Part print with two shaded views. Sizes in mm from the minimum x, y, z corner. A direction names the side the tool comes from. Round coordinates to 2 decimals unless told otherwise and drop trailing zeros. Write each loop counter-clockwise with the first axis right and the second up, starting at its lowest first coordinate (ties: lowest second). Pieces come first, ordered by that corner, then holes. Notation, with made-up numbers: (11.5, 48.5) -> (15.5, 48.5) arc R26 cw to (15.5, 73.5) -> close; hole circle Ø8 at (26, 30). An arc over 180 degrees is marked (long way). Return JSON: item names as keys, results as strings. Group by question number.
(1) Saw through at A-A (x = 5). List the corners of the cut face in (y, z).
(2) Saw through at C-C (z = 17.35). List the corners of the cut face in (x, y), plus the area to 3 significant figures.
(3) Saw through at D-D (x = 18). List the corners of the cut face in (y, z).
(4) Saw through at B-B (z = 3.1). List the corners of the cut face in (x, y), plus the area to 3 significant figures.
(5) Drop flat-ended pins along their axis: pin 1 Ø10 at (x, z) = (15.5, 30.5) entering from +Y; pin 2 Ø8 at (y, z) = (23, 27.5) entering from -X; pin 3 Ø4 at (x, y) = (10, 33.5) entering from +Z; pin 4 Ø3.5 at (x, z) = (10, 5) entering from +Y. Give the stop position or say it passes through.
(6) Drill centre lines: L1, parallel to Z at x = 5, y = 28.25; L2, parallel to X at y = 28, z = 51; L3, parallel to Y at x = 16.5, z = 16.5. Where is each one in solid material? Low to high. Write a range as from..to.
(7) Tool access for the marked faces 1, 2 and 3: list every direction of +Z, -Z, +X, -X, +Y, -Y with a clear straight run to the whole face (end or side of a thin tool).
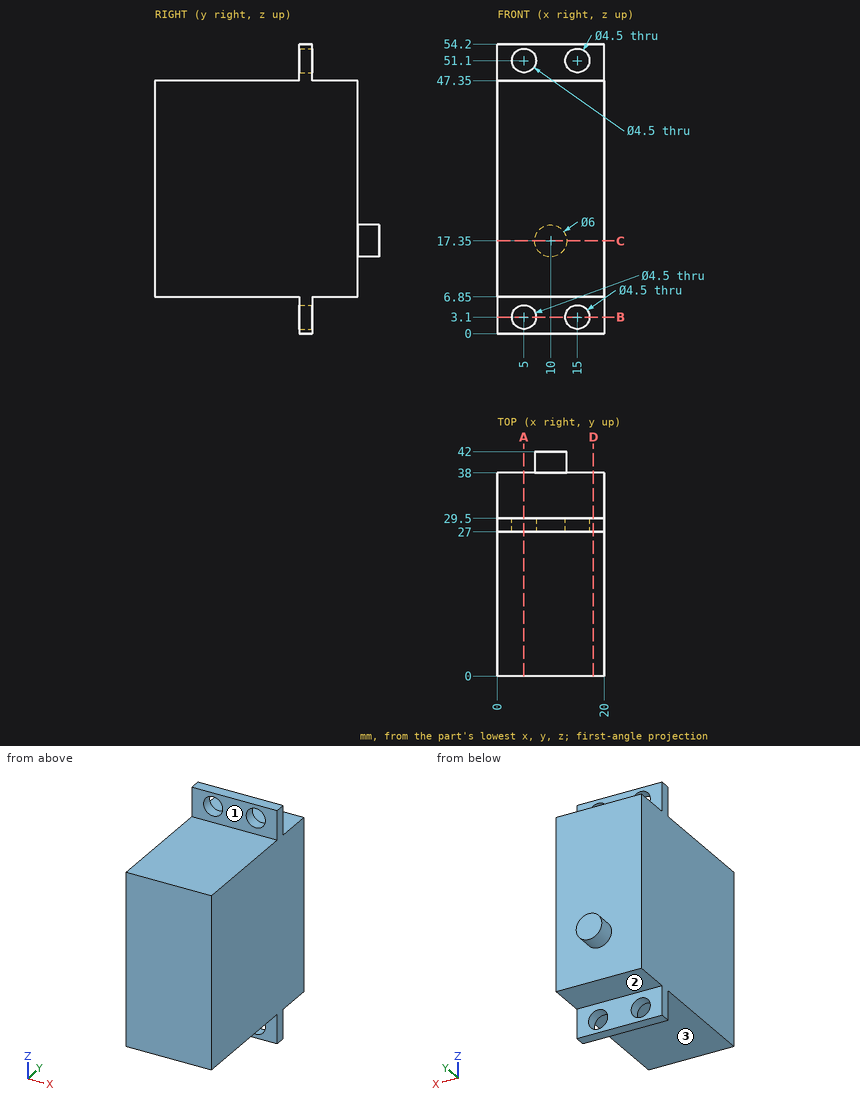
Computed values:
{
 "1": {"outline": "(0, 6.85) -> (27, 6.85) -> (27, 5.35) -> (29.5, 5.35) -> (29.5, 6.85) -> (38, 6.85) -> (38, 47.35) -> (29.5, 47.35) -> (29.5, 48.85) -> (27, 48.85) -> (27, 47.35) -> (0, 47.35) -> close; (27, 0) -> (29.5, 0) -> (29.5, 0.85) -> (27, 0.85) -> close; (27, 53.35) -> (29.5, 53.35) -> (29.5, 54.2) -> (27, 54.2) -> close"},
 "2": {"outline": "(0, 0) -> (20, 0) -> (20, 38) -> (13, 38) -> (13, 42) -> (7, 42) -> (7, 38) -> (0, 38) -> close", "area": "784 mm2"},
 "3": {"outline": "(0, 6.85) -> (27, 6.85) -> (27, 0) -> (29.5, 0) -> (29.5, 6.85) -> (38, 6.85) -> (38, 47.35) -> (29.5, 47.35) -> (29.5, 54.2) -> (27, 54.2) -> (27, 47.35) -> (0, 47.35) -> close"},
 "4": {"outline": "(0, 27) -> (2.75, 27) -> (2.75, 29.5) -> (0, 29.5) -> close; (7.25, 27) -> (12.75, 27) -> (12.75, 29.5) -> (7.25, 29.5) -> close; (17.25, 27) -> (20, 27) -> (20, 29.5) -> (17.25, 29.5) -> close", "area": "27.5 mm2"},
 "5": {"pin 1": "y = 38", "pin 2": "x = 0", "pin 3": "z = 47.35", "pin 4": "y = 29.5"},
 "6": {"L1": "0..0.85, 5.35..48.85, 53.35..54.2", "L2": "0..2.75, 7.25..12.75, 17.25..20", "L3": "0..38"},
 "7": {"face 1": "+Z, +X, -X, -Y", "face 2": "-Z, +X, -X, +Y", "face 3": "-Z, +X, -X, -Y"}
}
